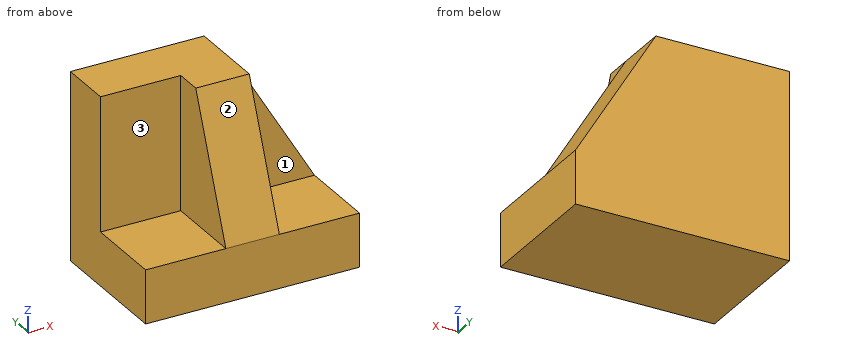
from build123d import *

# Parameters (mm, degrees)
F0_W     = 50.8
F0_H     = 44.45
F1_DEPTH = 31.75
F2_W     = 19.05
F2_H     = 31.75
F3_DEPTH = 19.05
F5_DEPTH = 12.7
F7_DEPTH = 12.7
F8_W     = 19.05
F8_H     = 31.75
F9_DEPTH = 19.05


with BuildPart() as f1:
    # F0 (on Front) → F1 (new body)
    with BuildSketch(Plane.XZ):
        with Locations((-44.0256018192, 39.4437830464)):
            Rectangle(F0_W, F0_H)
    extrude(amount=F1_DEPTH)

    # F2 (on face) → F3 (cut)
    with BuildSketch(Plane.YZ.offset(-18.6256018192)):
        with Locations((-22.225, 45.7937830464)):
            Rectangle(F2_W, F2_H)
    extrude(amount=-F3_DEPTH, mode=Mode.SUBTRACT)

    # F4 (on face) → F5 (cut)
    with BuildSketch(Plane(origin=(0, 0, 0), x_dir=(-1, 0, 0), z_dir=(0, 1, 0))):
        Polygon((18.6256018192, 29.9187830464), (37.6756018192, 61.6687830464), (18.6256018192, 61.6687830464), align=None)
    extrude(amount=-F5_DEPTH, mode=Mode.SUBTRACT)

    # F6 (on face) → F7 (cut)
    with BuildSketch(Plane.YZ.offset(-37.6756018192)):
        Polygon((-31.75, 29.9187830464), (-19.05, 61.6687830464), (-31.75, 61.6687830464), align=None)
    extrude(amount=-F7_DEPTH, mode=Mode.SUBTRACT)

    # F8 (on face) → F9 (cut)
    with BuildSketch(Plane(origin=(-69.4256018192, 0, 0), x_dir=(0, -1, 0), z_dir=(-1, 0, 0))):
        with Locations((22.225, 45.7937830464)):
            Rectangle(F8_W, F8_H)
    extrude(amount=-F9_DEPTH, mode=Mode.SUBTRACT)


solid = f1.part
Can you work these out from the model? Positions are in its coordinate system, mm. Face numbers are marked on the shaded views. A direction names the side the tool comes from. Round coordinates to 2 decimals unless told otherwise and drop trailing zeros. Order: outer loops, then holes, each group sorted by start corner. A loop starts at its lowest first (then second) coordinate and runs counter-clockwise, first axis right, second up. Notation, with made-up numbers: (-34, 72) - (18, 72) arc R18 ccw to (18, 79) - close; hole circle Ø6 at (11.25, -30.5). An arc over 180 degrees is marked (long way). Answer in a Markdown table with one row per item.
(1) Suppose I cut it at B-B, the plane y = -18. Please give me the cut outline in (x, z).
From the geometry:
| item | result |
|---|---|
| outline | (-69.43, 17.22) - (-18.63, 17.22) - (-18.63, 29.92) - (-37.68, 29.92) - (-37.68, 61.67) - (-50.38, 61.67) - (-50.38, 29.92) - (-69.43, 29.92) - close |
(2) Suppose I cut it at C-C, the plane z = 55. Please give me the cut outline in (x, y).
From the geometry:
| item | result |
|---|---|
| outline | (-69.43, -12.7) - (-50.38, -12.7) - (-50.38, -21.72) - (-37.68, -21.72) - (-37.68, -12.7) - (-33.67, -12.7) - (-33.67, 0) - (-69.43, 0) - close |
(3) Which directions (+Z, -Z, +X, -X, +Y, -Y) give clear straight access to the entire face, cutting with the end or side of a thin tool? Please do the marked faces 1, 2 and 3.
From the geometry:
| item | result |
|---|---|
| face 1 | +Z, +X, -Y |
| face 2 | +Z, +X, -X, -Y |
| face 3 | +Z, -X, -Y |
(4) For P1, Ø5.5, axis at y = -25.5, z = 38.5, coming from the +X side; P2, Ø9.5, axis at x = -63.5, y = -21.5, coming from the +Z side; P3, Ø4, axis at x = -35.5, z = 53.5, coming from the -Y side, each with a flat end and sliding along its axis, tell me the tip position at first contact or that it passes through.
From the geometry:
| item | result |
|---|---|
| P1 | stops at x = -37.68 |
| P2 | stops at z = 29.92 |
| P3 | stops at y = -12.7 |
(5) Suppose I cut it at A-A, the plane x = -42. Please give me the cut outline in (y, z).
From the geometry:
| item | result |
|---|---|
| outline | (-31.75, 17.22) - (0, 17.22) - (0, 61.67) - (-19.05, 61.67) - (-31.75, 29.92) - close |
(6) Suppose I cut it at D-D, the plane x = -59. Please give me the cut outline in (y, z), plus the area to 3 significant figures.
From the geometry:
| item | result |
|---|---|
| outline | (-31.75, 17.22) - (0, 17.22) - (0, 61.67) - (-12.7, 61.67) - (-12.7, 29.92) - (-31.75, 29.92) - close |
| area | 806 mm2 |
(7) Please list where these lines run through material, in increasing order: L1, parallel to Z at x = -54, y = -21.5; L2, parallel to X at y = -14, z = 32.5; L3, parallel to Y at x = -31.5, z = 38.5. Write a range as from..to.
From the geometry:
| item | result |
|---|---|
| L1 | z = 17.22..29.92 |
| L2 | x = -50.38..-37.68 |
| L3 | y = -12.7..0 |
